The model under review builds one solid part; all positions refer to its coordinate system, in mm. A direction names the side the tool comes from. Give positions to 0.01 mm unless a question says otherwise; leave off trailing zeros. Loops run counter-clockwise (first coordinate to the right, second up) from the corner with the lowest first, then second, coordinate; pieces in that order, holes last. Notation, with made-up numbers: M 56,36 L 98,36 A25 cw 98,51 Z; hole C 16,-38 d10. An arc over 180 degrees is marked long. Return JSON: item names as keys, results as strings. Group by question number.
```python
from build123d import *

# Parameters (mm, degrees)
BOSS_EXTRUDE1_DEPTH = 2


with BuildPart() as part:
    # Sketch2 → Revolve1 (revolve)
    with BuildSketch(Plane.XY):
        Polygon((2.475, 2), (2.475, 1.2), (1.245, 1.2), (1.245, 0.45), (2.375, 0.45), (2.375, -2), (3.535, -2), (3.535, 2), align=None)
    revolve(axis=Axis((0, 55, 0), (0, -1, 0)))

    # Sketch3 → Boss-Extrude1 (add)
    with BuildSketch(Plane(origin=(0, 0, 0), x_dir=(1, 0, 0), z_dir=(0, 1, 0))):
        with BuildLine():
            ThreePointArc((3.535, 0), (3.180996027, -1.541910917), (2.189885842, -2.775))
            Line((2.189885842, -2.775), (14.232465575, -1.773881029))
            ThreePointArc((14.232465575, -1.773881029), (13.044016702, -1.443867644), (12.3554, -0.420575606))
            ThreePointArc((12.3554, -0.420575606), (11.845417029, -0.438862165), (11.585, 0))
            Line((11.585, 0), (10.585, 0))
            ThreePointArc((10.585, 0), (10.085, -0.5), (9.585, 0))
            Line((9.585, 0), (8.585, 0))
            ThreePointArc((8.585, 0), (8.085, -0.5), (7.585, 0))
            Line((7.585, 0), (6.585, 0))
            ThreePointArc((6.585, 0), (6.085, -0.5), (5.585, 0))
            Line((5.585, 0), (4.585, 0))
            ThreePointArc((4.585, 0), (4.085, -0.5), (3.585, 0))
            Line((3.585, 0), (3.535, 0))
        make_face()
        with BuildLine():
            ThreePointArc((12.3554, -0.420575606), (13.044016702, -1.443867644), (14.232465575, -1.773881029))
            ThreePointArc((14.232465575, -1.773881029), (15.394749733, -1.205386095), (15.865, 0))
            Line((15.865, 0), (14.585, 0))
            ThreePointArc((14.585, 0), (14.085, -0.5), (13.585, 0))
            Line((13.585, 0), (12.585, 0))
            ThreePointArc((12.585, 0), (12.523862165, -0.239582971), (12.3554, -0.420575606))
        make_face()
    boss_extrude1 = extrude(amount=BOSS_EXTRUDE1_DEPTH)

    # Mirror1: Boss-Extrude1 across plane
    add(boss_extrude1.mirror(Plane(origin=(0, 15.95383002, 0), x_dir=(1, 0, 0), z_dir=(0, 0, -1))))


solid = part.part
```
(1) For probe 1 along Y at (x, z) = (3.75, -1); probe 2 along Z at (x, y) = (0, 1.8) (3 decimals); probe 3 along X at (y, z) = (0.75, -1), list the stretches that pass through material, from the lowest coordinate up.
(2) For faces 4 (the cylindrical face through (2.36, 1.59, 0.74)), 5 (the cylindrical face through (3.688, 0.986, 0.304)), 6 (the flat face through (-1, 0.45, -1)), list the 3-axis set-ups (+Z, -Z, +X, -X, +Y, -Y) from which the entire face can be reached by the end or side of a thin tool; tool diameter is ignored.
(3) Add section D-D (z = 2). Write out the cut boundary in (x, y).
(4) For pin 1 (3 mm diameter, centred on x = 0, z = 0, fed in from -Y); pin 2 (1 mm diameter, centred on x = 10, z = -1, fed in from -Y); pin 3 (3 mm diameter, centred on x = 0, z = 0, fed in from +Y), all flat-tipped, find the tip position at first contact; note any pin that passes through.
(5) Add section B-B (y = 1.65). Write out the cut boundary in (x, z) (3 decimals), and give its area (3 significant figures).
(6) Add section A-A (x = -0.25). Write out the cut boundary in (y, z), and give its area (3 significant figures).
(7) Add section C-C (z = -0.75). Write out the cut boundary in (x, y).
(8) Mouldability with a two-part tool opening along X and no side actions: class faces 1 (the flat face through (6, 2, -1)), 2 (the flat face through (8.13, 0.99, -2.28)), 3 (the cylindrical face through (14.56, 0.99, -0.15)) as released by +X, released by -X, zero draft, split by the parting line, or undercut.
Verdict:
{
 "1": {"probe 1": "y = 0 to 2", "probe 2": "z = -3.535 to -2.475, 2.475 to 3.535", "probe 3": "x = -3.39 to -0.74, 0.74 to 15.56"},
 "2": {"face 4": "+Y", "face 5": "+Y, -Y", "face 6": "-Y"},
 "3": {"outline": "M -2.91,-2 L -1.28,-2 L -1.28,0.45 L 1.28,0.45 L 1.28,-2 L 2.91,-2 L 2.91,0 L 11.51,0 L 11.51,2 L 1.46,2 L 1.46,1.2 L -1.46,1.2 L -1.46,2 L -2.91,2 Z"},
 "4": {"pin 1": "stops at y = 0.45", "pin 2": "stops at y = 0", "pin 3": "stops at y = 1.2"},
 "5": {"outline": "M 2.19,-2.775 L 14.232,-1.774 A1.78 ccw 14.232,1.774 L 2.19,2.775 A3.535 ccw long Z; hole C 0,0 d4.95; hole C 4.085,0 d1; hole C 6.085,0 d1; hole C 8.085,0 d1; hole C 10.085,0 d1; hole C 12.085,0 d1; hole C 14.085,0 d1", "area": "69.3 mm²"},
 "6": {"outline": "M -2,-3.53 L 2,-3.53 L 2,-2.46 L 1.2,-2.46 L 1.2,-1.22 L 0.45,-1.22 L 0.45,-2.36 L -2,-2.36 Z; M -2,2.36 L 0.45,2.36 L 0.45,1.22 L 1.2,1.22 L 1.2,2.46 L 2,2.46 L 2,3.53 L -2,3.53 Z", "area": "10.9 mm²"},
 "7": {"outline": "M -3.45,-2 L -2.25,-2 L -2.25,0.45 L -0.99,0.45 L -0.99,1.2 L -2.36,1.2 L -2.36,2 L -3.45,2 Z; M 0.99,0.45 L 2.25,0.45 L 2.25,-2 L 3.45,-2 L 3.45,0 L 15.7,0 L 15.7,2 L 2.36,2 L 2.36,1.2 L 0.99,1.2 Z"},
 "8": {"face 1": "zero draft", "face 2": "released by +X", "face 3": "undercut"}
}
